Input: dimensioned drawing with shaded views. Units: mm. Origin: part minimum x, y, z. A direction names the side the tool comes from. Round coordinates to 2 decimals unless told otherwise and drop trailing zeros. Order: outer loops, then holes, each group sorted by start corner. A loop starts at its lowest first (then second) coordinate and runs counter-clockwise, first axis right, second up. Notation, with made-up numbers: M 82.5,40 L 134.5,40 A10 ccw 134.5,45 Z; hole C 41,-6.75 d8. An arc over 180 degrees is marked long. Put each result on its own line as item: value. Start each with the question number.
1) Draft query along X for the marked faces 1, 2 and 3. Return one class per face: pulls with the +X half, pulls with the -X half, needs draft (parallel to the pull), parting line crosses it, or undercut.
2) Section B-B, the plane z = 4.4. Return loops of the section in (x, y).
3) Section C-C, the plane z = 1.15. Return loops of the section in (x, y).
4) Section A-A, the plane y = 8. Return loops of the section in (x, z).
5) Section D-D, the plane y = 1.5. Return loops of the section in (x, z), then the cut area to 3 significant figures.
6) First-contact query: P1, Ø0.9, axis at y = 2, z = 2, coming from the +X side; P2, Ø5, axis at x = 27.5, y = 13.5, coming from the +Z side; P3, Ø1.8, axis at x = 15, z = 1, coming from the -Y side; P4, Ø2, axis at x = 30, y = 19, coming from the +Z side. Flat tips, straight axial feed; report the tip coordinate or a pass-through.
7) Access query for the marked faces 4, 5, 6, 7 and 8. Directions: +Z, -Z, +X, -X, +Y, -Y. A direction counts if a zero-diameter tool reaches every point of the face in a straight line with its end or side. Return the directions, or none.
8) Material intervals for probe 1 along X at (y, z) = (6.5, 1.35); probe 2 along X at (y, z) = (10, 0.65); probe 3 along Z at (x, y) = (16, 12), sorted ascending. Write a range as [from, to].
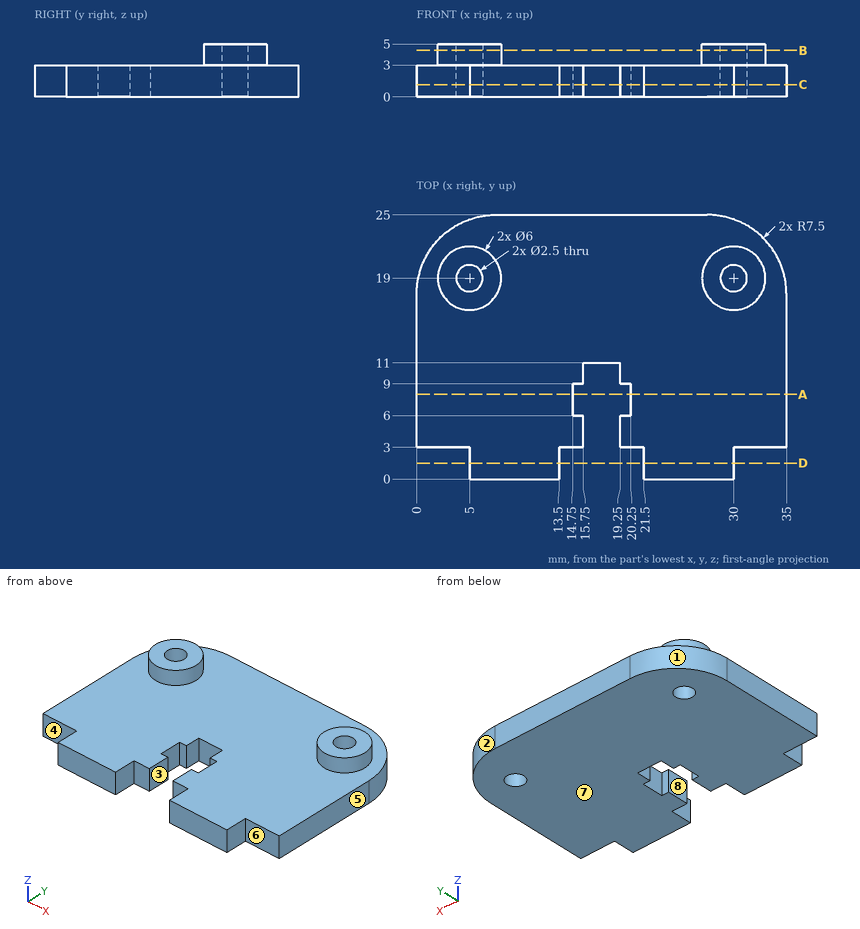
Result sheet:
1. face 1: pulls with the -X half
1. face 2: pulls with the +X half
1. face 3: undercut
2. outline: C 5,19 d6; C 30,19 d6; hole C 5,19 d2.5; hole C 30,19 d2.5
3. outline: M 0,3 L 5,3 L 5,0 L 13.5,0 L 13.5,3 L 15.75,3 L 15.75,6 L 14.75,6 L 14.75,9 L 15.75,9 L 15.75,11 L 19.25,11 L 19.25,9 L 20.25,9 L 20.25,6 L 19.25,6 L 19.25,3 L 21.5,3 L 21.5,0 L 30,0 L 30,3 L 35,3 L 35,17.5 A7.5 ccw 27.5,25 L 7.5,25 A7.5 ccw 0,17.5 Z; hole C 5,19 d2.5; hole C 30,19 d2.5
4. outline: M 0,0 L 14.75,0 L 14.75,3 L 0,3 Z; M 20.25,0 L 35,0 L 35,3 L 20.25,3 Z
5. outline: M 5,0 L 13.5,0 L 13.5,3 L 5,3 Z; M 21.5,0 L 30,0 L 30,3 L 21.5,3 Z
5. area: 51.0 mm2
6. P1: stops at x = 30
6. P2: stops at z = 3
6. P3: stops at y = 3
6. P4: passes through
7. face 4: +Z, -Z, -X, -Y
7. face 5: +Z, -Z, +X, +Y, -Y
7. face 6: +Z, -Z, +X, -Y
7. face 7: -Z, +X, -X, +Y, -Y
7. face 8: +Z, -Z, -Y
8. probe 1: x = [0, 14.75], [20.25, 35]
8. probe 2: x = [0, 15.75], [19.25, 35]
8. probe 3: z = [0, 3]
